Geometry check sheet. Reference: the model listing, model coordinates, mm. A direction names the side the tool comes from. Give positions to 0.01 mm unless a question says otherwise; leave off trailing zeros. Order: outer loops, then holes, each group sorted by start corner. A loop starts at its lowest first (then second) coordinate and runs counter-clockwise, first axis right, second up. Notation, with made-up numbers: M 57.5,24.5 L 73.5,24.5 A16 cw 73.5,48.5 Z; hole C 26,59 d4. An arc over 180 degrees is marked long. Put each result on its own line as item: value. Start each with the question number.
Q1. Mould release check, pull along Y, two halves, no side actions. Record for faces 6 (the cylindrical face through (2.198, 63.823, -3.314)), 7 (the cylindrical face through (-39.132, 79.273, -8.822)), 8 (the flat face through (1, 0, 15)), 9 (the flat face through (-50.8, 35, 8)): +Y half, -Y half, draft (parallel to the pull), parting line (faces both ways), or undercut.
Q2. Access from +Z, -Z, +X, -X, +Y, -Y to the whole of each face (thin tool, end or side, straight path). Record for faces 1 (the flat face through (-11, 61, -13.264)), 2 (the flat face through (25.4, 67, -5)), 3 (the flat face through (1, 15, 0)), 4 (the flat face through (-12.238, 27, 25)), 5 (the flat face through (50.8, 28, 13)).
Q3. Section check B-B on z = 26. Record the cut outline in (x, y).
Q4. Section check A-A on x = -38.1. Record the cut outline in (y, z).
Q5. Section check C-C on y = 15.5. Record the cut outline in (x, z), then the cut area to 3 significant figures.
Q6. Material ranges on L1, parallel to X at y = 21, z = 24; L2, parallel to Y at x = 0, z = -6; L3, parallel to Y at x = 33.5, z = 8, recorded low to high.
Q7. Go/stop test with flat-tipped pins: pin 1 (20.5 mm diameter, centred on x = 44, z = -2.5, fed in from +Y); pin 2 (12.5 mm diameter, centred on x = -38.1, y = 68.05, fed in from +Z); pin 3 (6.5 mm diameter, centred on x = 7.5, z = -5, fed in from -Y). Record where each tip stops, or that it passes through.
Q8. Section check D-D on x = 38. Record the cut outline in (y, z), then the cut area to 3 significant figures.
```python
from build123d import *

# Parameters (mm, degrees)
F1_DEPTH = 50.8
F3_DEPTH = 53.8666486626
F4_W     = 34.3918725848
F4_H     = 43.6418196186
F5_DEPTH = 25.4
F6_R     = 4.7625
F7_DEPTH = 50.8


with BuildPart() as f1:
    # F0 (on Right) → F1 (new body, symmetric)
    with BuildSketch(Plane.YZ):
        Polygon((0, 29.2371641845), (0, 0), (31.0912281275, 0), (31.0912281275, -13.2636902854), (91.8474793434, -13.2636902854), (43.3565787971, 29.2371641845), align=None)
    extrude(amount=F1_DEPTH, both=True)

    # F2 (on face) → F3 (cut, through all)
    with BuildSketch(Plane.XZ):
        Polygon((13.1616968006, 29.2371641845), (0, 29.2371641845), (-12.2383031994, 29.2371641845), (-12.2383031994, 20.0262721628), (13.1616968006, 20.0262721628), align=None)
    extrude(amount=-F3_DEPTH, mode=Mode.SUBTRACT)

    # F4 (on face) → F5 (cut)
    with BuildSketch(Plane.YZ.offset(50.8)):
        with Locations((74.651543051, 8.5572195239)):
            Rectangle(F4_W, F4_H)
    extrude(amount=-F5_DEPTH, mode=Mode.SUBTRACT)

    # F6 (on Top) → F7 (cut, symmetric)
    with BuildSketch(Plane.XY):
        with Locations((-38.1, 83.9226793434)):
            Circle(F6_R)
        with Locations((-38.1, 68.0476793434)):
            Circle(F6_R)
        with Locations((0, 83.9226793434)):
            Circle(F6_R)
        with Locations((0, 68.0476793434)):
            Circle(F6_R)
    extrude(amount=F7_DEPTH, both=True, mode=Mode.SUBTRACT)


solid = f1.part
```
Results found:
1. face 6: undercut
1. face 7: undercut
1. face 8: -Y half
1. face 9: draft
2. face 1: -Z, +X, -X, +Y, -Y
2. face 2: +Z, -Z, +X, +Y
2. face 3: -Z, +X, -X, -Y
2. face 4: +Z, +Y, -Y
2. face 5: +Z, -Z, +X, +Y, -Y
3. outline: M -50.8,0 L -12.24,0 L -12.24,47.05 L -50.8,47.05 Z; M 13.16,0 L 50.8,0 L 50.8,47.05 L 13.16,47.05 Z
4. outline: M 0,0 L 31.09,0 L 31.09,-13.26 L 63.29,-13.26 L 63.29,11.77 L 43.36,29.24 L 0,29.24 Z; M 72.81,-13.26 L 79.16,-13.26 L 79.16,-2.14 L 72.81,3.42 Z; M 88.69,-13.26 L 91.85,-13.26 L 88.69,-10.49 Z
5. outline: M -50.8,0 L 50.8,0 L 50.8,29.24 L 13.16,29.24 L 13.16,20.03 L -12.24,20.03 L -12.24,29.24 L -50.8,29.24 Z
5. area: 2,740 mm^2
6. L1: x = -50.8 to -12.24, 13.16 to 50.8
6. L2: y = 31.09 to 63.29, 72.81 to 79.16
6. L3: y = 0 to 57.46
7. pin 1: stops at y = 57.46
7. pin 2: stops at z = 13.07
7. pin 3: stops at y = 31.09
8. outline: M 0,0 L 31.09,0 L 31.09,-13.26 L 57.46,-13.26 L 57.46,16.88 L 43.36,29.24 L 0,29.24 Z
8. area: 1,940 mm^2
